CAD build for the part. Positions are in the model's coordinates, mm. Face numbers are marked on the shaded views. A direction names the side the tool comes from. Round coordinates to 2 decimals unless told otherwise and drop trailing zeros. Write each loop counter-clockwise with the first axis right and the second up, starting at its lowest first coordinate (ties: lowest second). Pieces come first, ordered by that corner, then holes. Notation, with made-up numbers: (17.25, -12) -> (58.25, -12) arc R16 ccw to (58.25, 10) -> close; hole circle Ø2 at (77.5, 41). An arc over 180 degrees is marked (long way). Put each result on its own line as item: value. Start each with the question number.
1. Pull direction X, two halves, no side cores. Call the marked faces 1, 2 and 3: pulls with the +X half, pulls with the -X half, needs draft (parallel to the pull), parting line crosses it, or undercut.
2. Saw through at D-D on y = -7.5. List the corners of the cut face in (x, z), and give its area (3 significant figures).
3. Flat gauge pins, fed straight in: P1, Ø2, axis at x = -1.5, z = 4, coming from the -Y side; P2, Ø2, axis at y = 3, z = -16, coming from the -X side; P3, Ø8, axis at y = 2, z = -10, coming from the -X side; P4, Ø3.5, axis at x = 0, y = 0, coming from the +Z side. Where does each tip first touch, or does it go through?
4. Saw through at B-B on x = 0. List the corners of the cut face in (y, z).
5. Saw through at A-A on z = 0. List the corners of the cut face in (x, y).
6. Saw through at C-C on y = 0. List the corners of the cut face in (x, z), and give its area (3 significant figures).
7. Drill centre lines: line 1 (X direction, y = 5.25, z = 0); line 2 (X direction, y = 0, z = -22.4); line 3 (Z direction, x = -12, y = -7.25). Where is each one in solid material? Low to high. Write a range as from..to.
8. 3-axis set-ups, long thin cutter, end or side, ignore diameter. For the marked faces 4 and 5: which of +Z, -Z, +X, -X, +Y, -Y reach the whole face in a straight line?
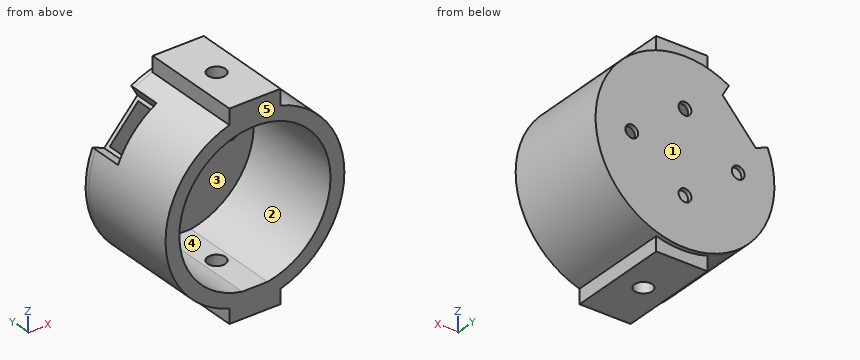
from build123d import *
from build123d.topology import SkipClean

# Parameters (mm, degrees)
SKETCH1_R           = 21
SKETCH1_R_2         = 17.75
BOSS_EXTRUDE2_DEPTH = 12
SKETCH5_W           = 12
SKETCH5_H           = 6
BOSS_EXTRUDE7_DEPTH = 12
SKETCH6_W           = 12
SKETCH6_H           = 6
BOSS_EXTRUDE8_DEPTH = 12
SKETCH7_R           = 2.1
CUT_EXTRUDE1_DEPTH  = 54.080717
BOSS_EXTRUDE9_START = 1
SKETCH8_R           = 21
BOSS_EXTRUDE9_DEPTH = 1
CUT_EXTRUDE2_REACH  = 42.374
SKETCH9_R           = 1.5
CUT_EXTRUDE6_START  = 5
CUT_EXTRUDE6_DEPTH  = 30.264595


with BuildPart() as part:
    # Sketch1 → Boss-Extrude2 (new, symmetric)
    with BuildSketch(Plane(origin=(0, 0, 0), x_dir=(1, 0, 0), z_dir=(0, 1, 0))):
        with Locations(Location((0, 0, 0), (0, 0, 270))):
            Circle(SKETCH1_R)
        with Locations(Location((0, 0, 0), (0, 0, 270))):
            Circle(SKETCH1_R_2, mode=Mode.SUBTRACT)
    extrude(amount=BOSS_EXTRUDE2_DEPTH, both=True)

    # Sketch6 → Boss-Extrude8 (add, symmetric)
    with BuildSketch(Plane(origin=(0, 0, 0), x_dir=(1, 0, 0), z_dir=(0, 1, 0))):
        with Locations((0, -20.75)):
            Rectangle(SKETCH6_W, SKETCH6_H)
    extrude(amount=BOSS_EXTRUDE8_DEPTH, both=True)


with BuildPart() as body_2:
    # Sketch5 → Boss-Extrude7 (new, symmetric)
    with BuildSketch(Plane(origin=(0, 0, 0), x_dir=(1, 0, 0), z_dir=(0, 1, 0))):
        with Locations((0, 20.5)):
            Rectangle(SKETCH5_W, SKETCH5_H)
    extrude(amount=BOSS_EXTRUDE7_DEPTH, both=True)


with BuildPart() as cut_extrude1_tool:
    # Sketch7 → Cut-Extrude1 (new, through all)
    with BuildSketch(Plane(origin=(0, 0, -23.5), x_dir=(-1, 0, 0), z_dir=(0, 0, -1))):
        Circle(SKETCH7_R)
    extrude(amount=-CUT_EXTRUDE1_DEPTH)


with BuildPart() as part_1:
    add(part.part)

    # Cut-Extrude1: cut by cut_extrude1_tool
    add(cut_extrude1_tool.part, mode=Mode.SUBTRACT)



with BuildPart() as body_2_1:
    add(body_2.part)

    # Cut-Extrude1: cut by cut_extrude1_tool
    add(cut_extrude1_tool.part, mode=Mode.SUBTRACT)


with BuildPart() as part_2:
    with SkipClean():  # the faces are left unmerged after this step: merging them gives an invalid solid
        add(part_1.part)

        add(body_2_1.part)  # Boss-Extrude9 merges body 2
        # Sketch8 → Boss-Extrude9 (add)
        with BuildSketch(Plane(origin=(0, 12, 0), x_dir=(1, 0, 0), z_dir=(0, 1, 0)).offset(BOSS_EXTRUDE9_START)):
            with Locations(Location((0, 0, 0), (0, 0, 106.60155))):
                Circle(SKETCH8_R)
        extrude(amount=-BOSS_EXTRUDE9_DEPTH)

    # Sketch9 → Cut-Extrude2 (cut, up to next)
    with BuildSketch(Plane(origin=(0, 13, 0), x_dir=(1, 0, 0), z_dir=(0, 1, 0)), mode=Mode.PRIVATE) as cut_extrude2_sk1:
        with Locations(Location((0, 9.5, 0), (0, 0, 270))):
            Circle(SKETCH9_R)
    cut_extrude2_tool1 = extrude(cut_extrude2_sk1.sketch, amount=-CUT_EXTRUDE2_REACH, mode=Mode.PRIVATE) & part_2.part
    # Sketch9 → Cut-Extrude2 (cut, up to next)
    with BuildSketch(Plane(origin=(0, 13, 0), x_dir=(1, 0, 0), z_dir=(0, 1, 0)), mode=Mode.PRIVATE) as cut_extrude2_sk2:
        with Locations(Location((0, -9.5, 0), (0, 0, 270))):
            Circle(SKETCH9_R)
    cut_extrude2_tool2 = extrude(cut_extrude2_sk2.sketch, amount=-CUT_EXTRUDE2_REACH, mode=Mode.PRIVATE) & part_2.part
    # Sketch9 → Cut-Extrude2 (cut, up to next)
    with BuildSketch(Plane(origin=(0, 13, 0), x_dir=(1, 0, 0), z_dir=(0, 1, 0)), mode=Mode.PRIVATE) as cut_extrude2_sk3:
        with Locations(Location((-12.5, 0, 0), (0, 0, 270))):
            Circle(SKETCH9_R)
    cut_extrude2_tool3 = extrude(cut_extrude2_sk3.sketch, amount=-CUT_EXTRUDE2_REACH, mode=Mode.PRIVATE) & part_2.part
    # Sketch9 → Cut-Extrude2 (cut, up to next)
    with BuildSketch(Plane(origin=(0, 13, 0), x_dir=(1, 0, 0), z_dir=(0, 1, 0)), mode=Mode.PRIVATE) as cut_extrude2_sk4:
        with Locations(Location((12.5, 0, 0), (0, 0, 270))):
            Circle(SKETCH9_R)
    cut_extrude2_tool4 = extrude(cut_extrude2_sk4.sketch, amount=-CUT_EXTRUDE2_REACH, mode=Mode.PRIVATE) & part_2.part
    add(cut_extrude2_tool1.solids().sort_by_distance((0, 13, -9.5))[0], mode=Mode.SUBTRACT)
    add(cut_extrude2_tool2.solids().sort_by_distance((0, 13, 9.5))[0], mode=Mode.SUBTRACT)
    add(cut_extrude2_tool3.solids().sort_by_distance((-12.5, 13, 0))[0], mode=Mode.SUBTRACT)
    add(cut_extrude2_tool4.solids().sort_by_distance((12.5, 13, 0))[0], mode=Mode.SUBTRACT)

    # Sketch12 → Cut-Extrude6 (cut, through all)
    with SkipClean():  # the faces are left unmerged after this step: merging them gives an invalid solid
        with BuildSketch(Plane(origin=(0, 0, 0), x_dir=(1, 0, 0), z_dir=(0, 1, 0)).offset(CUT_EXTRUDE6_START)):
            with BuildLine():
                Line((-19.403691, -8.030988), (-16.631735, -6.883704))
                Line((-16.631735, -6.883704), (-8.848918, -15.674714))
                Line((-8.848918, -15.674714), (-10.323738, -18.287166))
                ThreePointArc((-10.323738, -18.287166), (-15.723464, -13.920226), (-19.403691, -8.030988))
            make_face()
        extrude(amount=CUT_EXTRUDE6_DEPTH, mode=Mode.SUBTRACT)


solid = part_2.part
Return value:
1. face 1: needs draft
1. face 2: undercut
1. face 3: undercut
2. outline: (-6, -23.5) -> (6, -23.5) -> (6, -20.12) arc R21 ccw to (6, 20.12) -> (6, 23.75) -> (-6, 23.75) -> (-6, 20.12) arc R21 ccw to (-6, -20.12) -> close; hole (-2.97, -17.5) -> (2.97, -17.5) arc R17.75 ccw (long way) to start
2. area: 467 mm^2
3. P1: stops at y = 12
3. P2: stops at x = -14.7
3. P3: stops at x = -20.12
3. P4: passes through
4. outline: (-12, -23.5) -> (-2.1, -23.5) -> (-2.1, -17.5) -> (-12, -17.5) -> close; (-12, 17.75) -> (-2.1, 17.75) -> (-2.1, 23.75) -> (-12, 23.75) -> close; (2.1, -23.5) -> (12, -23.5) -> (12, -21) -> (13, -21) -> (13, -11) -> (12, -11) -> (12, -17.5) -> (2.1, -17.5) -> close; (2.1, 17.75) -> (12, 17.75) -> (12, 11) -> (13, 11) -> (13, 21) -> (12, 21) -> (12, 23.75) -> (2.1, 23.75) -> close; (12, -8) -> (13, -8) -> (13, 8) -> (12, 8) -> close
5. outline: (-21, -12) -> (-17.75, -12) -> (-17.75, 12) -> (-14, 12) -> (-14, 13) -> (-21, 13) -> close; (-11, 12) -> (11, 12) -> (11, 13) -> (-11, 13) -> close; (14, 12) -> (17.75, 12) -> (17.75, -12) -> (21, -12) -> (21, 13) -> (14, 13) -> close
6. outline: (-6, -23.5) -> (-2.1, -23.5) -> (-2.1, -17.5) -> (-2.97, -17.5) arc R17.75 cw to (-2.1, 17.63) -> (-2.1, 23.75) -> (-6, 23.75) -> (-6, 20.12) arc R21 ccw to (-6, -20.12) -> close; (2.1, -23.5) -> (6, -23.5) -> (6, -20.12) arc R21 ccw to (6, 20.12) -> (6, 23.75) -> (2.1, 23.75) -> (2.1, 17.63) arc R17.75 cw to (2.97, -17.5) -> (2.1, -17.5) -> close
6. area: 416 mm^2
7. line 1: x = -21..-17.75, 17.75..21
7. line 2: x = -6..-2.1, 2.1..6
7. line 3: z = -17.23..-13.08, 13.08..17.23
8. face 4: -Y
8. face 5: +Z, -Z, +X, -X, -Y
